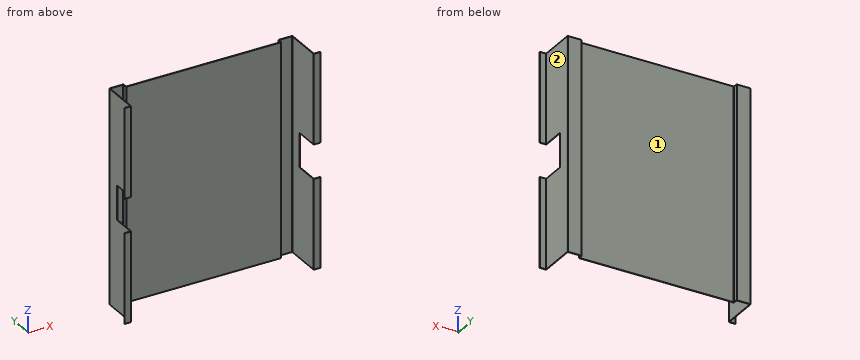
```python
from build123d import *

# Parameters (mm, degrees)
SKETCH_1_W             = 181
SKETCH_1_H             = 500
SM_BASE_FLANGE_1_DEPTH = 1
SM_EDGE_FLANGE_1_DEPTH = 500
SM_EDGE_FLANGE_2_DEPTH = 500
SM_EDGE_FLANGE_3_DEPTH = 500
SM_EDGE_FLANGE_4_DEPTH = 500
SKETCH_18_W            = 80
SKETCH_18_H            = 71.447403799
CUT_EXTRUDE_1_DEPTH    = 100


# Sheet-metal steps are written as plain solids
with BuildPart() as part:
    # Sketch 1 → 基体-法兰1 (new body)
    with BuildSketch(Plane(origin=(0, 0, 0), x_dir=(1, 0, 0), z_dir=(0, 1, 0))):
        with Locations((-90.5, 0)):
            Rectangle(SKETCH_1_W, SKETCH_1_H)
    extrude(amount=-SM_BASE_FLANGE_1_DEPTH)

    # 边线-法兰1 section (across the edge) → 边线-法兰1 (add)
    with BuildSketch(Plane(origin=(-181.5, 0, -250), x_dir=(1, 0, 0), z_dir=(0, 0, 1))):
        with BuildLine():
            Line((-1, 0.5), (-1, 9))
            Line((-1, 9), (0, 9))
            Line((0, 9), (0, 0.5))
            ThreePointArc((0, 0.5), (0.146446609, 0.146446609), (0.5, 0))
            Line((0.5, 0), (0.5, -1))
            ThreePointArc((0.5, -1), (-0.560660172, -0.560660172), (-1, 0.5))
        make_face()
    extrude(amount=SM_EDGE_FLANGE_1_DEPTH)

    # 边线-法兰2 section (across the edge) → 边线-法兰2 (add)
    with BuildSketch(Plane(origin=(-182.5, 9.5, 250), x_dir=(0, -1, 0), z_dir=(0, 0, -1))):
        with BuildLine():
            Line((-1, 0.5), (-1, 31))
            Line((-1, 31), (0, 31))
            Line((0, 31), (0, 0.5))
            ThreePointArc((0, 0.5), (0.146446609, 0.146446609), (0.5, 0))
            Line((0.5, 0), (0.5, -1))
            ThreePointArc((0.5, -1), (-0.560660172, -0.560660172), (-1, 0.5))
        make_face()
    extrude(amount=SM_EDGE_FLANGE_2_DEPTH)

    # 边线-法兰3 section (across the edge) → 边线-法兰3 (add)
    with BuildSketch(Plane(origin=(-214, 9.5, 250), x_dir=(1, 0, 0), z_dir=(0, 0, -1))):
        with BuildLine():
            Line((-1, 0.5), (-1, 84))
            Line((-1, 84), (0, 84))
            Line((0, 84), (0, 0.5))
            ThreePointArc((0, 0.5), (0.146446609, 0.146446609), (0.5, 0))
            Line((0.5, 0), (0.5, -1))
            ThreePointArc((0.5, -1), (-0.560660172, -0.560660172), (-1, 0.5))
        make_face()
    extrude(amount=SM_EDGE_FLANGE_3_DEPTH)

    # 边线-法兰4 section (across the edge) → 边线-法兰4 (add)
    with BuildSketch(Plane(origin=(-215, -75, -250), x_dir=(0, 1, 0), z_dir=(0, 0, 1))):
        with BuildLine():
            Line((-1, 0.5), (-1, 15))
            Line((-1, 15), (0, 15))
            Line((0, 15), (0, 0.5))
            ThreePointArc((0, 0.5), (0.146446609, 0.146446609), (0.5, 0))
            Line((0.5, 0), (0.5, -1))
            ThreePointArc((0.5, -1), (-0.560660172, -0.560660172), (-1, 0.5))
        make_face()
    extrude(amount=SM_EDGE_FLANGE_4_DEPTH)

    # 草图18 → 切除-拉伸1 (cut)
    with BuildSketch(Plane.ZY.offset(230)):
        with Locations((0, -55.723701899)):
            Rectangle(SKETCH_18_W, SKETCH_18_H)
    extrude(amount=-CUT_EXTRUDE_1_DEPTH, mode=Mode.SUBTRACT)

    # 镜向1: part across plane


with BuildPart() as part_1:
    add(part.part)
    add(part.part.mirror(Plane(origin=(0, -1, -250), x_dir=(0, 0, 1), z_dir=(1, 0, 0))))


solid = part_1.part
```
Here's how the part is built. I have some questions about the finished solid (model axes, mm). Face numbers are marked on the shaded views. Round coordinates to 2 decimals unless told otherwise and drop trailing zeros. Loops run counter-clockwise (first coordinate to the right, second up) from the corner with the lowest first, then second, coordinate; pieces in that order, holes last. Notation, with made-up numbers: (87.25, 27.25) -> (136.25, 27.25) arc R23 ccw to (136.25, 64.25) -> close; hole circle Ø4 at (-11.75, 29). An arc over 180 degrees is marked (long way). Answer as CSV lines item,"result".
1. For pin 1 (13 mm diameter, centred on x = 223, y = -38.5, fed in from -Z); pin 2 (0.8 mm diameter, centred on x = -214.5, z = 2, fed in from -Y); pin 3 (4.5 mm diameter, centred on x = -219.5, z = -126.5, fed in from +Y); pin 4 (5 mm diameter, centred on x = -165, z = -154.5, fed in from +Y), each with a flat end and sliding along its axis, tell me the tip position at first contact or that it passes through.
Final values:
pin 1,"passes through"
pin 2,"stops at y = -20"
pin 3,"stops at y = -75"
pin 4,"stops at y = 0"
2. If we section it at C-C on x = -36: Please give me the cut outline in (y, z).
Final values:
outline,"(-1, -250) -> (0, -250) -> (0, 250) -> (-1, 250) -> close"
3. If we section it at A-A on y = -35: Please give me the cut outline in (x, z), plus the area to 3 significant figures.
Final values:
outline,"(-215, -250) -> (-214, -250) -> (-214, -40) -> (-215, -40) -> close; (-215, 40) -> (-214, 40) -> (-214, 250) -> (-215, 250) -> close; (214, -250) -> (215, -250) -> (215, -40) -> (214, -40) -> close; (214, 40) -> (215, 40) -> (215, 250) -> (214, 250) -> close"
area,"840 mm^2"
4. If we section it at B-B on z = 16: Please give me the cut outline in (x, y), plus the area to 3 significant figures.
Final values:
outline,"(-215, -20) -> (-214, -20) -> (-214, 9) arc R0.5 cw to (-213.5, 9.5) -> (-183, 9.5) arc R0.5 cw to (-182.5, 9) -> (-182.5, 0.5) arc R1.5 ccw to (-181, -1) -> (181, -1) arc R1.5 ccw to (182.5, 0.5) -> (182.5, 9) arc R0.5 cw to (183, 9.5) -> (213.5, 9.5) arc R0.5 cw to (214, 9) -> (214, -20) -> (215, -20) -> (215, 9) arc R1.5 ccw to (213.5, 10.5) -> (183, 10.5) arc R1.5 ccw to (181.5, 9) -> (181.5, 0.5) arc R0.5 cw to (181, 0) -> (-181, 0) arc R0.5 cw to (-181.5, 0.5) -> (-181.5, 9) arc R1.5 ccw to (-183, 10.5) -> (-213.5, 10.5) arc R1.5 ccw to (-215, 9) -> close"
area,"507 mm^2"
5. If I drill on L1, parallel to X at y = -69.5, z = -155.5; L2, parallel to Y at x = 146.5, z = -218; L3, parallel to Y at x = -189, z = -71.5, over which ranges is the centre line in solid material (lowest first)?
Final values:
L1,"x = -215 to -214, 214 to 215"
L2,"y = -1 to 0"
L3,"y = 9.5 to 10.5"
6. Thinking about a two-plate mould opening in X: for the marked faces 1 and 2, which applies, released by +X, released by -X, zero draft, split by the parting line, or undercut?
Final values:
face 1,"undercut"
face 2,"released by +X"
